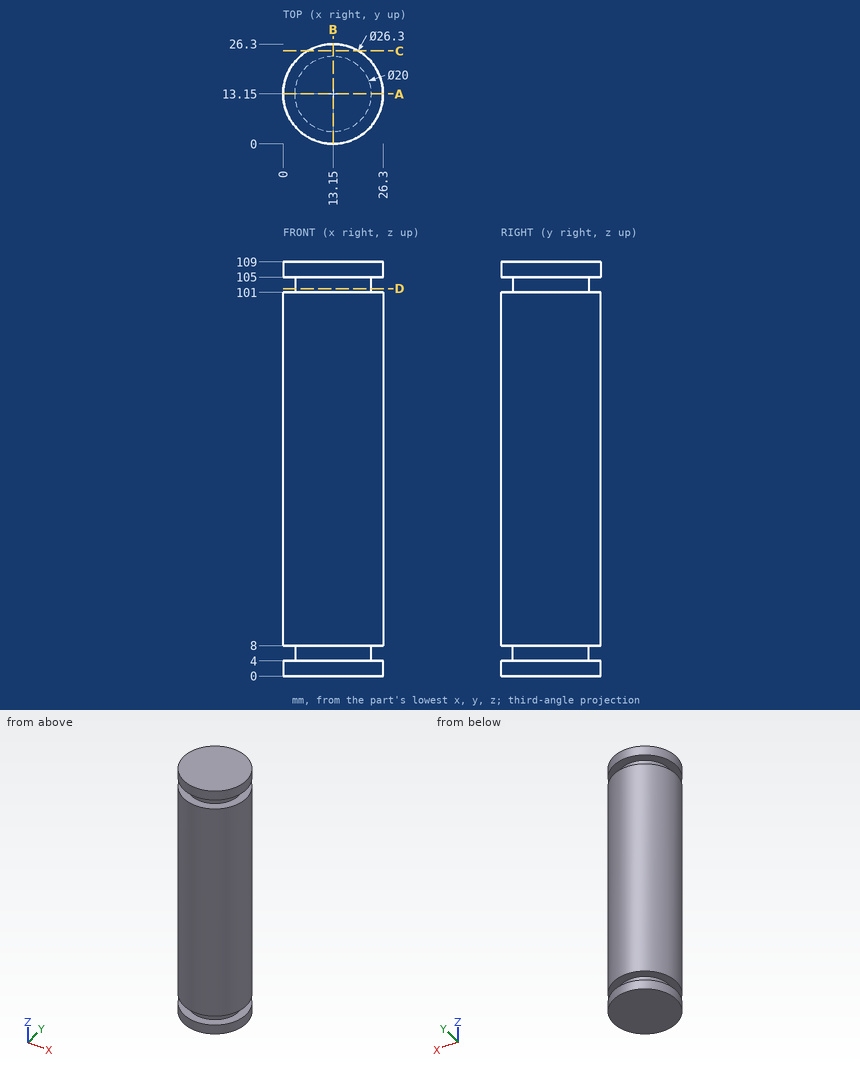
The figure shows three views and two pictorial views of one solid part (mm, origin at its lowest corner). Answer the questions. Round coordinates to 2 decimals unless told otherwise and drop trailing zeros. Write each loop counter-clockwise with the first axis right and the second up, starting at its lowest first coordinate (ties: lowest second). Pieces come first, ordered by that corner, then holes. Notation, with made-up numbers: (-17, 61.25) - (-5, 61.25) arc R21 ccw to (-5, 70.25) - close; hole circle Ø11 at (-7.5, 46). An arc over 180 degrees is marked (long way). Use one line per item in the form item = value. Start each with the question number.
Item 1: A cutting plane is placed at D-D (z = 102). Write down the section's boundary in (x, y), plus the area to 3 significant figures.
Item 2: A cutting plane is placed at A-A (y = 13.15). Write down the section's boundary in (x, z).
Item 3: Flat-ended cylindrical pins translate along their axes: pin 1 Ø12 at (y, z) = (5.5, 45) entering from +X; pin 2 Ø1 at (y, z) = (23, 72) entering from -X; pin 3 Ø5 at (x, z) = (18, 66.5) entering from -Y. Find the tip coordinate at first contact, or state that the pin passes through.
Item 4: Find the intervals of material crossed by line 1 (Z direction, x = 16.25, y = 23.75); line 2 (X direction, y = 14.25, z = 95.5); line 3 (Y direction, x = 3.75, z = 67), in increasing order. Write a range as [from, to].
Item 5: A cutting plane is placed at C-C (y = 24.5). Write down the section's boundary in (x, z).
The answers:
q1.outline = circle Ø20 at (13.15, 13.15)
q1.area = 314 mm^2
q2.outline = (0, 0) - (26.3, 0) - (26.3, 4) - (23.15, 4) - (23.15, 8) - (26.3, 8) - (26.3, 101) - (23.15, 101) - (23.15, 105) - (26.3, 105) - (26.3, 109) - (0, 109) - (0, 105) - (3.15, 105) - (3.15, 101) - (0, 101) - (0, 8) - (3.15, 8) - (3.15, 4) - (0, 4) - close
q3.pin_1 = 26.2
q3.pin_2 = 3.9
q3.pin_3 = 0.21
q4.line_1 = [0, 4], [8, 101], [105, 109]
q4.line_2 = [0.05, 26.25]
q4.line_3 = [3.95, 22.35]
q5.outline = (6.51, 0) - (19.79, 0) - (19.79, 4) - (6.51, 4) - close; (6.51, 8) - (19.79, 8) - (19.79, 101) - (6.51, 101) - close; (6.51, 105) - (19.79, 105) - (19.79, 109) - (6.51, 109) - close
